```python
from build123d import *

# Parameters (mm, degrees)
SZKIC1_R                    = 2.2
SZKIC1_R_2                  = 1
DODANIE_WYCI_GNI_CIE1_DEPTH = 4
SZKIC2_R                    = 5.75
SZKIC2_W                    = 4
SZKIC2_H                    = 34.7
WYTNIJ_WYCI_GNI_CIE1_DEPTH  = 3
SZKIC3_W                    = 5
SZKIC3_H                    = 2.8
SZKIC3_W_2                  = 8
SZKIC3_H_2                  = 10
SZKIC3_H_3                  = 7
DODANIE_WYCI_GNI_CIE2_DEPTH = 2.6
SZKIC4_R                    = 5.75
SZKIC4_W                    = 7
SZKIC4_H                    = 7
SZKIC4_R_2                  = 2.2
WYTNIJ_WYCI_GNI_CIE3_DEPTH  = 2


with BuildPart() as part:
    # Szkic1 → Dodanie-wyciągnięcie1 (new body)
    with BuildSketch(Plane.XY):
        Polygon((-39.75, -15.95), (-39.75, -18.75), (39.75, -18.75), (39.75, 18.75), (7.15, 18.75), (7.15, -15.95), align=None)
        with Locations((24.05, -9.85)):
            Circle(SZKIC1_R, mode=Mode.SUBTRACT)
        with Locations((16.55, 0.15)):
            Circle(SZKIC1_R, mode=Mode.SUBTRACT)
        with Locations((24.05, 0.15)):
            Circle(SZKIC1_R, mode=Mode.SUBTRACT)
        with Locations((31.55, 0.15)):
            Circle(SZKIC1_R, mode=Mode.SUBTRACT)
        with Locations((33.15, 9.15)):
            Circle(SZKIC1_R_2, mode=Mode.SUBTRACT)
        with Locations((24.05, 10.15)):
            Circle(SZKIC1_R, mode=Mode.SUBTRACT)
    extrude(amount=DODANIE_WYCI_GNI_CIE1_DEPTH)

    # Szkic2 → Wytnij-wyciągnięcie1 (cut)
    with BuildSketch(Plane(origin=(0, 0, 0), x_dir=(-1, 0, 0), z_dir=(0, 0, -1))):
        with Locations((-33.15, 9.15)):
            Circle(SZKIC2_R)
        with Locations((-9.15, 1.4)):
            Rectangle(SZKIC2_W, SZKIC2_H)
    extrude(amount=-WYTNIJ_WYCI_GNI_CIE1_DEPTH, mode=Mode.SUBTRACT)

    # Szkic3 → Dodanie-wyciągnięcie2 (add)
    with BuildSketch(Plane(origin=(0, 0, 0), x_dir=(-1, 0, 0), z_dir=(0, 0, -1))):
        with Locations((18.25, -17.35)):
            Rectangle(SZKIC3_W, SZKIC3_H)
        with Locations((-16.15, 12.75)):
            Rectangle(SZKIC3_W_2, SZKIC3_H_2)
        with Locations((-31.55, -11.35)):
            Rectangle(SZKIC3_W, SZKIC3_H_3)
    extrude(amount=DODANIE_WYCI_GNI_CIE2_DEPTH)

    # Szkic4 → Wytnij-wyciągnięcie3 (cut)
    # profile 1 of 9: a face of its own
    with BuildSketch(Plane(origin=(0, 0, 0), x_dir=(-1, 0, 0), z_dir=(0, 0, -1))):
        with BuildLine():
            Line((-27.55, 10.454798835), (-27.55, 13.65))
            Line((-27.55, 13.65), (-29.570544734, 13.65))
            ThreePointArc((-29.570544734, 13.65), (-28.290172085, 12.223202342), (-27.55, 10.454798835))
        make_face()
    # profile 2 of 9: a face of its own
    with BuildSketch(Plane(origin=(0, 0, 0), x_dir=(-1, 0, 0), z_dir=(0, 0, -1))):
        with BuildLine():
            Line((-27.55, 6.65), (-27.55, 7.845201165))
            ThreePointArc((-27.55, 7.845201165), (-27.727927326, 7.235939416), (-27.971921206, 6.65))
            Line((-27.971921206, 6.65), (-27.55, 6.65))
        make_face()
    # profile 3 of 9: a face of its own
    with BuildSketch(Plane(origin=(0, 0, 0), x_dir=(-1, 0, 0), z_dir=(0, 0, -1))):
        with Locations((-33.15, 9.15)):
            Circle(SZKIC4_R)
    # profile 4 of 9: a face of its own
    with BuildSketch(Plane(origin=(0, 0, 0), x_dir=(-1, 0, 0), z_dir=(0, 0, -1))):
        with Locations((-24.05, 10.15)):
            Rectangle(SZKIC4_W, SZKIC4_H)
        with Locations((-24.05, 10.15)):
            Circle(SZKIC4_R_2, mode=Mode.SUBTRACT)
    # profile 5 of 9: a face of its own
    with BuildSketch(Plane(origin=(0, 0, 0), x_dir=(-1, 0, 0), z_dir=(0, 0, -1))):
        with Locations((-24.05, 0.15)):
            Rectangle(SZKIC4_W, SZKIC4_H)
        with Locations((-24.05, 0.15)):
            Circle(SZKIC4_R_2, mode=Mode.SUBTRACT)
    # profile 6 of 9: a face of its own
    with BuildSketch(Plane(origin=(0, 0, 0), x_dir=(-1, 0, 0), z_dir=(0, 0, -1))):
        with Locations((-33.15, 9.15)):
            Circle(SZKIC4_R)
    # profile 7 of 9: a face of its own
    with BuildSketch(Plane(origin=(0, 0, 0), x_dir=(-1, 0, 0), z_dir=(0, 0, -1))):
        with Locations((-31.55, 0.15)):
            Rectangle(SZKIC4_W, SZKIC4_H)
        with Locations((-31.55, 0.15)):
            Circle(SZKIC4_R_2, mode=Mode.SUBTRACT)
    # profile 8 of 9: a face of its own
    with BuildSketch(Plane(origin=(0, 0, 0), x_dir=(-1, 0, 0), z_dir=(0, 0, -1))):
        with Locations((-16.55, 0.15)):
            Rectangle(SZKIC4_W, SZKIC4_H)
        with Locations((-16.55, 0.15)):
            Circle(SZKIC4_R_2, mode=Mode.SUBTRACT)
    # profile 9 of 9: a face of its own
    with BuildSketch(Plane(origin=(0, 0, 0), x_dir=(-1, 0, 0), z_dir=(0, 0, -1))):
        with Locations((-24.05, -9.85)):
            Rectangle(SZKIC4_W, SZKIC4_H)
        with Locations((-24.05, -9.85)):
            Circle(SZKIC4_R_2, mode=Mode.SUBTRACT)
    extrude(amount=-WYTNIJ_WYCI_GNI_CIE3_DEPTH, mode=Mode.SUBTRACT)


solid = part.part
```
Geometry check sheet. Reference: the model listing, model coordinates, mm. A direction names the side the tool comes from. Give positions to 0.01 mm unless a question says otherwise; leave off trailing zeros. Order: outer loops, then holes, each group sorted by start corner. A loop starts at its lowest first (then second) coordinate and runs counter-clockwise, first axis right, second up. Notation, with made-up numbers: (87.25, 57.25) -> (142.25, 57.25) arc R24 cw to (142.25, 93.25) -> close; hole circle Ø7 at (34.25, 39). An arc over 180 degrees is marked (long way). Write each question's results on one line, items separated by ' | '. Start each with the question number.
(1) Mould release check, pull along Y, two halves, no side actions. Record for faces 1 (the face through (34.05, -11, -1)), 2 (the face through (17, 3.65, 1)), 3 (the face through (32, -14.85, -1)): pulls with the +Y half, pulls with the -Y half, needs draft (parallel to the pull), parting line crosses it, or undercut.
(2) Sectioned sample at D-D (y = -9.85). Enter the section's corners in (x, z).
(3) Scan lines: line 1 (X direction, y = 0.15, z = 3.65); line 2 (X direction, y = 9.15, z = 1.2); line 3 (Y direction, x = 4, z = 1.25). Record each from-to range of solid material in increasing order.
(4) Access from +Z, -Z, +X, -X, +Y, -Y to the whole of each face (thin tool, end or side, straight path). Record for faces 4 (the face through (20.15, 13, -1)), 5 (the face through (16, 7.75, -1)), 6 (the face through (32, -7.85, -1)), 7 (the face through (27.55, -10, 1)), 8 (the face through (29.05, -11, -1)).
(5) Gauge pin test, flat ends, axial feed: P1, Ø1.3, axis at y = -17, z = -1, coming from the -X side; P2, Ø2, axis at x = 22.5, y = 0, coming from the -Z side; P3, Ø1.1, axis at y = 4.5, z = 3.5, coming from the -X side. Record the tip position at first contact, or that the pin passes through.
(6) Sectioned sample at C-C (y = 0.15). Give the number of separate pieces and of enclosed holes in the cut face, plus the area to 3 significant figures.
(7) Sectioned sample at B-B (z = -1). Enter the section's corners in (x, y), plus the area to 3 significant figures.
(8) Sectioned sample at A-A (x = 24.05). Enter the section's corners in (y, z), plus the area to 3 significant figures.
Answer below:
1) face 1: needs draft | face 2: undercut | face 3: pulls with the -Y half
2) outline: (7.15, 3) -> (11.15, 3) -> (11.15, 0) -> (20.55, 0) -> (20.55, 2) -> (21.85, 2) -> (21.85, 4) -> (7.15, 4) -> close; (26.25, 2) -> (27.55, 2) -> (27.55, 0) -> (29.05, 0) -> (29.05, -2.6) -> (34.05, -2.6) -> (34.05, 0) -> (39.75, 0) -> (39.75, 4) -> (26.25, 4) -> close
3) line 1: 7.15 to 14.35, 18.75 to 21.85, 26.25 to 29.35, 33.75 to 39.75 | line 2: 11.15 to 20.55, 38.9 to 39.75 | line 3: -18.75 to -15.95
4) face 4: -Z, +X, +Y, -Y | face 5: -Z, +X, -X, -Y | face 6: -Z, +X, -X, +Y | face 7: -Z | face 8: -Z, -X, +Y, -Y
5) P1: x = -20.75 | P2: z = 2 | P3: x = 7.15
6) separate pieces: 4 | enclosed holes: 0 | area: 50.0 mm2
7) outline: (-20.75, -18.75) -> (-15.75, -18.75) -> (-15.75, -15.95) -> (-20.75, -15.95) -> close; (12.15, 7.75) -> (20.15, 7.75) -> (20.15, 17.75) -> (12.15, 17.75) -> close; (29.05, -14.85) -> (34.05, -14.85) -> (34.05, -7.85) -> (29.05, -7.85) -> close | area: 129 mm2
8) outline: (-18.75, 0) -> (-13.35, 0) -> (-13.35, 2) -> (-12.05, 2) -> (-12.05, 4) -> (-18.75, 4) -> close; (-7.65, 2) -> (-6.35, 2) -> (-6.35, 0) -> (-3.35, 0) -> (-3.35, 2) -> (-2.05, 2) -> (-2.05, 4) -> (-7.65, 4) -> close; (2.35, 2) -> (3.65, 2) -> (3.65, 0) -> (6.65, 0) -> (6.65, 2) -> (7.95, 2) -> (7.95, 4) -> (2.35, 4) -> close; (12.35, 2) -> (13.65, 2) -> (13.65, 0) -> (18.75, 0) -> (18.75, 4) -> (12.35, 4) -> close | area: 81.6 mm2
